Work out the finished part from the listing and answer in its coordinate system (mm). Face numbers are marked on the shaded views. A direction names the side the tool comes from. Round coordinates to 2 decimals unless told otherwise and drop trailing zeros. Loops run counter-clockwise (first coordinate to the right, second up) from the corner with the lowest first, then second, coordinate; pieces in that order, holes last. Notation, with made-up numbers: M 18.25,76.25 L 31.25,76.25 A13 cw 31.25,80.25 Z; hole C -18,-10 d2. An arc over 180 degrees is marked long. One line per item, written item: value.
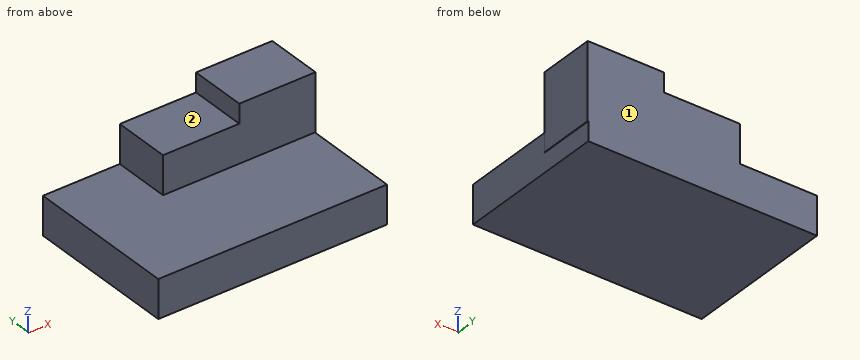
```python
from build123d import *

# Parameters (mm, degrees)
F0_W     = 152.4
F0_H     = 101.6
F1_DEPTH = 12.7
F2_W     = 50.8
F2_H     = 38.1
F3_DEPTH = 50.8
F4_DEPTH = 38.1


with BuildPart() as f1:
    # F0 (on Top) → F1 (new body, symmetric)
    with BuildSketch(Plane.XY):
        with Locations((14.2702582896, -2.3004743776)):
            Rectangle(F0_W, F0_H)
    extrude(amount=F1_DEPTH, both=True)

    # F2 (on Top) → F3 (join)
    with BuildSketch(Plane.XY):
        with Locations((65.439629665, 29.4495256224)):
            Rectangle(F2_W, F2_H)
    extrude(amount=F3_DEPTH)

    # F2 (on Top) → F4 (join)
    with BuildSketch(Plane.XY):
        with Locations((14.639629665, 29.4495256224)):
            Rectangle(F2_W, F2_H)
    extrude(amount=F4_DEPTH)


solid = f1.part
```
1) Find section B-B (x = 20). Give the vertices of the cut face in (y, z).
Check values:
outline: M -53.1,-12.7 L 48.5,-12.7 L 48.5,38.1 L 10.4,38.1 L 10.4,12.7 L -53.1,12.7 Z
2) Find section A-A (y = 26.5). Give the vertices of the cut face in (x, z).
Check values:
outline: M -61.93,-12.7 L 90.47,-12.7 L 90.47,0 L 90.84,0 L 90.84,50.8 L 40.04,50.8 L 40.04,38.1 L -10.76,38.1 L -10.76,12.7 L -61.93,12.7 Z
3) Each of these flat-tipped pins is pushed along its axis until it touches: pin 1 (12.5 mm diameter, centred on y = -20.5, z = -1, fed in from +X); pin 2 (4 mm diameter, centred on y = 12.5, z = 44, fed in from -X); pin 3 (10 mm diameter, centred on x = -35, y = -14, fed in from +Z); pin 4 (8 mm diameter, centred on y = -35.5, z = 14.5, fed in from -X). Where does it stop, or does it pass through?
Check values:
pin 1: x = 90.47
pin 2: x = 40.04
pin 3: z = 12.7
pin 4: x = -61.93
4) Find the intervals of material crossed by probe 1 along Z at (x, y) = (37, -14.5); probe 2 along Z at (x, y) = (15, 14); probe 3 along Y at (x, z) = (20.5, 34), in increasing order. Write a range as from..to.
Check values:
probe 1: -12.7..12.7
probe 2: -12.7..38.1
probe 3: 10.4..48.5
5) For the marked faces 1 and 2, determine the directions among +Z, -Z, +X, -X, +Y, -Y from which every point of the face is accessible in a straight line to the end or side of a thin tool.
Check values:
face 1: +Z, -Z, +X, -X, +Y
face 2: +Z, -X, +Y, -Y
6) Find section C-C (z = 44). Give the vertices of the cut face in (x, y).
Check values:
outline: M 40.04,10.4 L 90.84,10.4 L 90.84,48.5 L 40.04,48.5 Z
7) Find section D-D (x = -15). Give the vertices of the cut face in (y, z), then the cut area to 3 significant figures.
Check values:
outline: M -53.1,-12.7 L 48.5,-12.7 L 48.5,12.7 L -53.1,12.7 Z
area: 2,580 mm2
